Input: part model. Units: mm. Frame: model coordinates. Round coordinates to 2 decimals unless told otherwise and drop trailing zeros. Order: outer loops, then holes, each group sorted by start corner. A loop starts at its lowest first (then second) coordinate and runs counter-clockwise, first axis right, second up. Notation, with made-up numbers: (47, -19.75) - (76, -19.75) arc R34 cw to (76, 10.25) - close; hole circle Ø10 at (51, 66). An arc over 180 degrees is marked (long way). One line per item, written item: value. Start each with the question number.
from build123d import *

# Parameters (mm, degrees)
F0_R     = 10
F0_R_2   = 4
F1_DEPTH = 20
F3_DEPTH = 12.5


with BuildPart() as f1:
    # F0 (on Top) → F1 (new body)
    with BuildSketch(Plane.XY):
        with BuildLine():
            ThreePointArc((2.083333, -12.325166), (9.547033, -8.068715), (12.5, 0))
            ThreePointArc((12.5, 0), (9.547033, 8.068715), (2.083333, 12.325166))
            ThreePointArc((2.083333, 12.325166), (-12.5, 0), (2.083333, -12.325166))
        make_face()
        Circle(F0_R, mode=Mode.SUBTRACT)
        with BuildLine():
            ThreePointArc((37.5, 0), (35.72822, 4.841229), (31.25, 7.3951))
            ThreePointArc((31.25, 7.3951), (22.5, 0), (31.25, -7.3951))
            ThreePointArc((31.25, -7.3951), (35.72822, -4.841229), (37.5, 0))
        make_face()
        with Locations((30, 0)):
            Circle(F0_R_2, mode=Mode.SUBTRACT)
        with BuildLine():
            ThreePointArc((2.083333, 12.325166), (9.547033, 8.068715), (12.5, 0))
            ThreePointArc((12.5, 0), (9.547033, -8.068715), (2.083333, -12.325166))
            Line((2.083333, -12.325166), (31.25, -7.3951))
            ThreePointArc((31.25, -7.3951), (22.5, 0), (31.25, 7.3951))
            Line((31.25, 7.3951), (2.083333, 12.325166))
        make_face()
    extrude(amount=F1_DEPTH)

    # F2 (on Front) → F3 (cut, symmetric)
    with BuildSketch(Plane.XZ):
        Polygon((43.665298, 20), (7.017286, 20), (43.665298, 6.661214), align=None)
    extrude(amount=F3_DEPTH, both=True, mode=Mode.SUBTRACT)


solid = f1.part
Item 1: Section query B-B on z = 3.5. Return loops of the section in (x, y), and give its area (3 significant figures).
Item 2: Pull-direction query (Y, two-part tool) for faces 1 (the face through (16.871, 9.826, 7.638)), 2 (the face through (-2.17, -9.76, 9.86)), 3 (the face through (12, 0, 0)), 4 (the face through (16.462, -9.895, 7.638)); classes: released by +Y, released by -Y, zero draft, split by the parting line, or undercut.
Item 3: Section query D-D on y = 8.75. Return loops of the section in (x, z), and give its area (3 significant figures).
Item 4: Section query C-C on y = -2.25. Return loops of the section in (x, z), and give its area (3 significant figures).
Item 5: Line query: L1, parallel to X at y = -3, z = 3.5; L2, parallel to Y at x = 30, z = 8.75; L3, parallel to Y at x = -7, z = 14.75. Output: solid intervals per line, ascending.
Item 6: First-contact query: pin 1 Ø3 at (x, z) = (-3, 15) entering from -Y; pin 2 Ø6 at (x, z) = (30.5, 10) entering from +Y; pin 3 Ø1 at (x, y) = (16, 10) entering from -Z; pin 4 Ø1 at (x, z) = (-4.5, 9.5) entering from -Y. Flat tips, straight axial feed; report the tip coordinate or a pass-through.
Item 7: Section query A-A on x = 0. Return loops of the section in (y, z).
Geometry results:
1. outline: (2.08, -12.33) - (31.25, -7.4) arc R7.5 ccw to (31.25, 7.4) - (2.08, 12.33) arc R12.5 ccw (long way) to start; hole circle Ø20 at (0, 0); hole circle Ø8 at (30, 0)
1. area: 578 mm^2
2. face 1: released by +Y
2. face 2: undercut
2. face 3: zero draft
2. face 4: released by -Y
3. outline: (-8.93, 0) - (-4.84, 0) - (-4.84, 20) - (-8.93, 20) - close; (4.84, 0) - (23.23, 0) - (23.23, 14.1) - (7.02, 20) - (4.84, 20) - close
3. area: 402 mm^2
4. outline: (-12.3, 0) - (-9.74, 0) - (-9.74, 20) - (-12.3, 20) - close; (9.74, 0) - (26.69, 0) - (26.69, 12.84) - (9.74, 19.01) - close; (33.31, 0) - (37.15, 0) - (37.15, 9.03) - (33.31, 10.43) - close
4. area: 358 mm^2
5. L1: x = -12.13 to -9.54, 9.54 to 27.35, 32.65 to 36.87
5. L2: y = -7.61 to -4, 4 to 7.61
5. L3: y = -10.36 to -7.14, 7.14 to 10.36
6. pin 1: stops at y = -12.41
6. pin 2: stops at y = 8.03
6. pin 3: stops at z = 0
6. pin 4: stops at y = -11.84
7. outline: (-12.5, 0) - (-10, 0) - (-10, 20) - (-12.5, 20) - close; (10, 0) - (12.5, 0) - (12.5, 20) - (10, 20) - close
